Part model, mm, in its own coordinate system. Give positions to 0.01 mm unless a question says otherwise; leave off trailing zeros. Order: outer loops, then holes, each group sorted by start corner. A loop starts at its lowest first (then second) coordinate and runs counter-clockwise, first axis right, second up. Notation, with made-up numbers: (35, -30.5) - (67, -30.5) arc R22 cw to (67, -19.5) - close; hole circle Ø7 at (18, -7). An arc over 180 degrees is marked (long way). One line per item, written item: value.
```python
from build123d import *

# Parameters (mm, degrees)
F0_W     = 615.95
F0_H     = 76.2
F1_DEPTH = 231.775
F2_W     = 609.6
F2_H     = 228.6
F3_DEPTH = 76.201
F4_R     = 2.4765
F5_DEPTH = 615.951


with BuildPart() as f1:
    # F0 (on Top) → F1 (new body)
    with BuildSketch(Plane.XY):
        Rectangle(F0_W, F0_H)
    extrude(amount=F1_DEPTH)

    # F2 (on face) → F3 (cut, through all)
    with BuildSketch(Plane.XZ.offset(38.1)):
        with Locations((0, 114.3)):
            Rectangle(F2_W, F2_H)
    extrude(amount=-F3_DEPTH, mode=Mode.SUBTRACT)

    # F4 (on face) → F5 (cut, through all)
    with BuildSketch(Plane.YZ.offset(307.975)):
        with BuildLine():
            ThreePointArc((-27.8765, 38.1), (-25.4, 35.6235), (-22.9235, 38.1))
            ThreePointArc((-22.9235, 38.1), (-25.4, 40.5765), (-27.8765, 38.1))
        make_face()
        with Locations((25.4, 38.1)):
            Circle(F4_R)
    extrude(amount=-F5_DEPTH, mode=Mode.SUBTRACT)


solid = f1.part
```
1) Wall check: line 1 along Y through (x, z) = (306, 38); line 2 along X through (y, z) = (-16, 59) (3 decimals); line 3 along Z through (x, y) = (-305.95, -25.4) (1 decimal). Give the ranges that are in metal, low to high. Write a range as [from, to].
Answer:
line 1: y = [-38.1, -27.87], [-22.93, 22.93], [27.87, 38.1]
line 2: x = [-307.975, -304.8], [304.8, 307.975]
line 3: z = [0, 35.6], [40.6, 231.8]
2) Slice it at C-C on x = -105. Write the cut outline in (y, z) (3 decimals).
Answer:
outline: (-38.1, 228.6) - (38.1, 228.6) - (38.1, 231.775) - (-38.1, 231.775) - close
3) Drop flat-ended pins along their axis: P1, Ø4, axis at y = 25.4, z = 38.1, coming from the -X side; P2, Ø4, axis at x = -214, y = 23, coming from the -Z side. Give the stop position or say it passes through.
Answer:
P1: passes through
P2: stops at z = 228.6
4) Slice it at A-A on z = 174.5. Write the cut outline in (x, y) (3 decimals), then the cut area to 3 significant figures.
Answer:
outline: (-307.975, -38.1) - (-304.8, -38.1) - (-304.8, 38.1) - (-307.975, 38.1) - close; (304.8, -38.1) - (307.975, -38.1) - (307.975, 38.1) - (304.8, 38.1) - close
area: 484 mm2
5) Two-plate mould, pull along X, no slides. Class faces 1 (the face through (307.975, -1, 114)), 2 (the face through (-4, 1, 231.775)), 3 (the face through (-4, -1, 228.6)), 4 (the face through (-307.975, -1, 114)): pulls with the +X half, pulls with the -X half, needs draft (parallel to the pull), parting line crosses it, or undercut.
Answer:
face 1: pulls with the +X half
face 2: needs draft
face 3: undercut
face 4: pulls with the -X half
6) Slice it at B-B on y = -7.5. Write the cut outline in (x, z) (3 decimals), then the cut area to 3 significant figures.
Answer:
outline: (-307.975, 0) - (-304.8, 0) - (-304.8, 228.6) - (304.8, 228.6) - (304.8, 0) - (307.975, 0) - (307.975, 231.775) - (-307.975, 231.775) - close
area: 3,410 mm2
